Verification items for the finished model (mm, model axes). A direction names the side the tool comes from. Round coordinates to 2 decimals unless told otherwise and drop trailing zeros. Order: outer loops, then holes, each group sorted by start corner. A loop starts at its lowest first (then second) coordinate and runs counter-clockwise, first axis right, second up. Notation, with made-up numbers: (-14.5, 43) -> (1.5, 43) arc R28 ccw to (1.5, 61) -> close; hole circle Ø3 at (-19, 52). An arc over 180 degrees is marked (long way). Put each result on its own line as item: value.
from build123d import *

# Parameters (mm, degrees)
SKETCH1_W           = 80
SKETCH1_H           = 30
BOSS_EXTRUDE1_DEPTH = 20
CHAMFER1_SIZE       = 15
CHAMFER1_SIZE2      = 25.980762114
SKETCH2_W           = 43
SKETCH2_H           = 15
BOSS_EXTRUDE2_DEPTH = 30
CUT_EXTRUDE1_REACH  = 75.891
CUT_EXTRUDE2_DEPTH  = 3
SKETCH5_W           = 12
SKETCH5_H           = 12
BOSS_EXTRUDE3_DEPTH = 15
CHAMFER2_SIZE       = 12
CUT_EXTRUDE3_REACH  = 75.103
SKETCH6_R           = 2.6
SKETCH7_R           = 5.5
CUT_EXTRUDE4_DEPTH  = 20
CHAMFER3_SIZE       = 15
CHAMFER3_SIZE_2     = 25.980762114


# Some blends are built 0.0001 mm under size
with BuildPart() as part:
    # Sketch1 → Boss-Extrude1 (new body)
    with BuildSketch(Plane(origin=(0, 0, 0), x_dir=(0, 0, -1), z_dir=(1, 0, 0))):
        Rectangle(SKETCH1_W, SKETCH1_H)
    extrude(amount=-BOSS_EXTRUDE1_DEPTH)

    # Chamfer1
    chamfer1_edges = [part.edges().sort_by_distance(p)[0] for p in [
        (-10, -15, 40),
    ]]
    chamfer1_side = [part.faces().sort_by_distance(p)[0] for p in [
        (-10, -15, 0),
    ]]
    chamfer(chamfer1_edges, length=CHAMFER1_SIZE, length2=CHAMFER1_SIZE2, reference=chamfer1_side[0])

    # Sketch2 → Boss-Extrude2 (add)
    with BuildSketch(Plane(origin=(0, -14.575317547, 25.245190528), x_dir=(1, 0, 0), z_dir=(0, -0.5000000000000012, 0.866025403784438))):
        with Locations((-10.5, 7.009618943)):
            Rectangle(SKETCH2_W, SKETCH2_H)
    extrude(amount=BOSS_EXTRUDE2_DEPTH)

    # Sketch3 → Cut-Extrude1 (cut, up to next)
    with BuildSketch(Plane(origin=(0, 12.565698604, 7.254809472), x_dir=(1, 0, 0), z_dir=(0, 0.8660254037844378, 0.5000000000000013)), mode=Mode.PRIVATE) as cut_extrude1_sk1:
        with BuildLine():
            Line((-24.78, -34.150635095), (-24.78, -54.150635095))
            ThreePointArc((-24.78, -54.150635095), (-26.33, -55.700635095), (-27.88, -54.150635095))
            Line((-27.88, -54.150635095), (-27.88, -34.150635095))
            ThreePointArc((-27.88, -34.150635095), (-26.33, -32.600635095), (-24.78, -34.150635095))
        make_face()
    cut_extrude1_tool1 = extrude(cut_extrude1_sk1.sketch, amount=-CUT_EXTRUDE1_REACH, mode=Mode.PRIVATE) & part.part
    # Sketch3 → Cut-Extrude1 (cut, up to next)
    with BuildSketch(Plane(origin=(0, 12.565698604, 7.254809472), x_dir=(1, 0, 0), z_dir=(0, 0.8660254037844378, 0.5000000000000013)), mode=Mode.PRIVATE) as cut_extrude1_sk2:
        with BuildLine():
            Line((-2.94, -34.150635095), (-2.94, -54.150635095))
            ThreePointArc((-2.94, -54.150635095), (-4.49, -55.700635095), (-6.04, -54.150635095))
            Line((-6.04, -54.150635095), (-6.04, -34.150635095))
            ThreePointArc((-6.04, -34.150635095), (-4.49, -32.600635095), (-2.94, -34.150635095))
        make_face()
    cut_extrude1_tool2 = extrude(cut_extrude1_sk2.sketch, amount=-CUT_EXTRUDE1_REACH, mode=Mode.PRIVATE) & part.part
    add(cut_extrude1_tool1.solids().sort_by_distance((-26.33, -9.509619, 45.490381))[0], mode=Mode.SUBTRACT)
    add(cut_extrude1_tool2.solids().sort_by_distance((-4.49, -9.509619, 45.490381))[0], mode=Mode.SUBTRACT)

    # Sketch4 → Cut-Extrude2 (cut)
    with BuildSketch(Plane(origin=(0, -0.424682453, -0.245190528), x_dir=(1, 0, 0), z_dir=(0, -0.8660254037844379, -0.5000000000000013))):
        with BuildLine():
            Line((-23.58, 54.150635095), (-23.58, 34.150635095))
            ThreePointArc((-23.58, 34.150635095), (-26.33, 31.400635095), (-29.08, 34.150635095))
            Line((-29.08, 34.150635095), (-29.08, 54.150635095))
            ThreePointArc((-29.08, 54.150635095), (-26.33, 56.900635095), (-23.58, 54.150635095))
        make_face()
        with BuildLine():
            Line((-1.74, 54.150635095), (-1.74, 34.150635095))
            ThreePointArc((-1.74, 34.150635095), (-4.49, 31.400635095), (-7.24, 34.150635095))
            Line((-7.24, 34.150635095), (-7.24, 54.150635095))
            ThreePointArc((-7.24, 54.150635095), (-4.49, 56.900635095), (-1.74, 54.150635095))
        make_face()
    extrude(amount=-CUT_EXTRUDE2_DEPTH, mode=Mode.SUBTRACT)

    # Sketch5 → Boss-Extrude3 (add)
    with BuildSketch(Plane(origin=(0, 12.565698604, 7.254809472), x_dir=(1, 0, 0), z_dir=(0, 0.8660254037844378, 0.5000000000000013))):
        with Locations((-26, -23.150635095)):
            Rectangle(SKETCH5_W, SKETCH5_H)
    extrude(amount=-BOSS_EXTRUDE3_DEPTH)

    # Chamfer2
    chamfer2_edges = [part.edges().sort_by_distance(p)[0] for p in [
        (-32, -2.504809472, 18.357695155),
    ]]
    chamfer(chamfer2_edges, length=CHAMFER2_SIZE - 0.0001)  # a hair under: the kernel refuses the full size

    # Sketch6 → Cut-Extrude3 (cut, up to next)
    with BuildSketch(Plane.XZ.offset(15), mode=Mode.PRIVATE) as cut_extrude3_sk1:
        with Locations(Location((-10, -30, 0), (0, 0, 270))):
            Circle(SKETCH6_R)
    cut_extrude3_tool1 = extrude(cut_extrude3_sk1.sketch, amount=-CUT_EXTRUDE3_REACH, mode=Mode.PRIVATE) & part.part
    # Sketch6 → Cut-Extrude3 (cut, up to next)
    with BuildSketch(Plane.XZ.offset(15), mode=Mode.PRIVATE) as cut_extrude3_sk2:
        with Locations(Location((-10, -15, 0), (0, 0, 270))):
            Circle(SKETCH6_R)
    cut_extrude3_tool2 = extrude(cut_extrude3_sk2.sketch, amount=-CUT_EXTRUDE3_REACH, mode=Mode.PRIVATE) & part.part
    # Sketch6 → Cut-Extrude3 (cut, up to next)
    with BuildSketch(Plane.XZ.offset(15), mode=Mode.PRIVATE) as cut_extrude3_sk3:
        with Locations(Location((-10, 0, 0), (0, 0, 270))):
            Circle(SKETCH6_R)
    cut_extrude3_tool3 = extrude(cut_extrude3_sk3.sketch, amount=-CUT_EXTRUDE3_REACH, mode=Mode.PRIVATE) & part.part
    # Sketch6 → Cut-Extrude3 (cut, up to next)
    with BuildSketch(Plane.XZ.offset(15), mode=Mode.PRIVATE) as cut_extrude3_sk4:
        with Locations(Location((-10, 15, 0), (0, 0, 270))):
            Circle(SKETCH6_R)
    cut_extrude3_tool4 = extrude(cut_extrude3_sk4.sketch, amount=-CUT_EXTRUDE3_REACH, mode=Mode.PRIVATE) & part.part
    add(cut_extrude3_tool1.solids().sort_by_distance((-10, -15, -30))[0], mode=Mode.SUBTRACT)
    add(cut_extrude3_tool2.solids().sort_by_distance((-10, -15, -15))[0], mode=Mode.SUBTRACT)
    add(cut_extrude3_tool3.solids().sort_by_distance((-10, -15, 0))[0], mode=Mode.SUBTRACT)
    add(cut_extrude3_tool4.solids().sort_by_distance((-10, -15, 15))[0], mode=Mode.SUBTRACT)

    # Sketch7 → Cut-Extrude4 (cut)
    with BuildSketch(Plane.XZ.offset(15)):
        with Locations(Location((-10, 15, 0), (0, 0, 270))):
            Circle(SKETCH7_R)
        with Locations(Location((-10, 0, 0), (0, 0, 270))):
            Circle(SKETCH7_R)
        with Locations(Location((-10, -15, 0), (0, 0, 270))):
            Circle(SKETCH7_R)
        with Locations(Location((-10, -30, 0), (0, 0, 270))):
            Circle(SKETCH7_R)
    extrude(amount=-CUT_EXTRUDE4_DEPTH, mode=Mode.SUBTRACT)

    # Chamfer3
    # the kernel refuses this chamfer: 25.980762114, 15 mm, written as the material it takes off along each edge
    with BuildSketch(Plane(origin=(67.214459559, -15, -40), x_dir=(0, 0.9983227437537926, -0.057893862402671366), z_dir=(-1, 0, 0))) as chamfer3_piece_1:
        Polygon((CHAMFER3_SIZE * 0.998322743754, -CHAMFER3_SIZE * 0.0578938624027), (-CHAMFER3_SIZE_2 * 0.0578938624016, -CHAMFER3_SIZE_2 * 0.998322743736), (0, 0), align=None)
    extrude(amount=154.428919118, mode=Mode.SUBTRACT)


solid = part.part
Item 1: Gauge pin test, flat ends, axial feed: pin 1 Ø3.5 at (x, z) = (-12.5, -29) entering from -Y; pin 2 Ø1.5 at (x, y) = (1.5, -17.5) entering from -Z; pin 3 Ø12 at (x, z) = (-4.5, 44) entering from -Y; pin 4 Ø4.5 at (x, z) = (-10, -30) entering from -Y. Record the tip position at first contact, or that the pin passes through.
Check sheet entries:
pin 1: stops at y = 5
pin 2: stops at z = 28.03
pin 3: stops at y = -29.43
pin 4: passes through
Item 2: Material ranges on L1, parallel to X at y = -19.5, z = 35.5; L2, parallel to X at y = -20, z = 42; L3, parallel to X at y = -4, z = -15, recorded low to high. Write a range as [from, to].
Check sheet entries:
L1: x = [-32, -29.08], [-23.58, -7.24], [-1.74, 11]
L2: x = [-32, -27.88], [-24.78, -6.04], [-2.94, 11]
L3: x = [-20, -15.5], [-4.5, 0]
Item 3: Section check A-A on z = 0. Record the boundary of the cut face in (x, y).
Check sheet entries:
outline: (-20, -15) -> (-15.5, -15) -> (-15.5, 5) -> (-12.6, 5) -> (-12.6, 15) -> (-20, 15) -> close; (-7.4, 5) -> (-4.5, 5) -> (-4.5, -15) -> (0, -15) -> (0, 15) -> (-7.4, 15) -> close
Item 4: Section check B-B on y = 6. Record the boundary of the cut face in (x, z), then the cut area to 3 significant figures.
Check sheet entries:
outline: (-20, -40) -> (0, -40) -> (0, 37.12) -> (-20, 37.12) -> close; hole circle Ø5.2 at (-10, -30); hole circle Ø5.2 at (-10, -15); hole circle Ø5.2 at (-10, 0); hole circle Ø5.2 at (-10, 15)
area: 1,460 mm^2
Item 5: Release check for a two-part mould opening along Y. For faces 1 (the flat face through (-5, 15, 1)), 2 (the flat face through (-11, 5, 18)), 3 (the flat face through (-9.86, 4.577, 36.302)), 4 (the cylindrical face through (-11.582, 9.93, -27.937)) record: +Y half, -Y half, draft (parallel to the pull), parting line (faces both ways), or undercut.
Check sheet entries:
face 1: +Y half
face 2: -Y half
face 3: undercut
face 4: draft
Item 6: Section check C-C on z = -15. Record the boundary of the cut face in (x, y).
Check sheet entries:
outline: (-20, -14.43) -> (-15.5, -14.43) -> (-15.5, 5) -> (-12.6, 5) -> (-12.6, 15) -> (-20, 15) -> close; (-7.4, 5) -> (-4.5, 5) -> (-4.5, -14.43) -> (0, -14.43) -> (0, 15) -> (-7.4, 15) -> close
Item 7: Tool access check on faces 5 (the flat face through (-10, 13, 40)), 6 (the flat face through (-10, -15, 6)), 7 (the flat face through (-6.28, -19.99, 39.64)), 8 (the flat face through (5.423, -8.414, 28.802)). Record the directions out of +Z, -Z, +X, -X, +Y, -Y that give a thin tool (end or side, any length) a straight path to the whole face; none if there is none.
Check sheet entries:
face 5: +Z, +X, -X, +Y
face 6: -Z, +X, -X, -Y
face 7: none
face 8: -Z, +X, +Y
Item 8: Section check D-D on x = -10. State how many separate pieces and enclosed holes the cut face has, then the cut area to 3 significant figures.
Check sheet entries:
separate pieces: 5
enclosed holes: 0
area: 1,490 mm^2
